```python
from build123d import *

# Parameters (mm, degrees)
BOSS_EXTRUDE3_DEPTH = 150
SKETCH3_W           = 5
SKETCH3_H           = 300
BOSS_EXTRUDE4_DEPTH = 194.04


with BuildPart() as part:
    # Sketch1 → Boss-Extrude3 (new, symmetric)
    with BuildSketch(Plane.XY):
        Polygon((-605.658970563, 869.326926327), (-605.421491465, 714.331361266), (-602.421487943, 714.331361266), (-602.651320044, 864.335957761), (-602.656320364, 867.599518288), (-455.616774381, 952.797835671), (-452.784185512, 951.168221277), (-322.765615027, 876.367343414), (-321.26959747, 878.967714824), (-451.288167955, 953.768592687), (-455.622120304, 956.261955282), align=None)
    extrude(amount=BOSS_EXTRUDE3_DEPTH, both=True)

    # Sketch3 → Boss-Extrude4 (add)
    with BuildSketch(Plane(origin=(-529.334093448, 913.551431111, 0), x_dir=(0.8652472150761933, 0.5013454465764019, 0), z_dir=(-0.5013454465764018, 0.8652472150761932, 0))):
        with Locations((62.691806295, 0)):
            Rectangle(SKETCH3_W, SKETCH3_H)
        with Locations((-65.711641465, 0)):
            Rectangle(SKETCH3_W, SKETCH3_H)
    extrude(amount=BOSS_EXTRUDE4_DEPTH)


solid = part.part
```
Design review of the part built by this model. Coordinates are the model's own, in mm. A direction names the side the tool comes from. Coordinates: 2 decimals unless noted, no trailing zeros. Loops run counter-clockwise (first coordinate to the right, second up) from the corner with the lowest first, then second, coordinate; pieces in that order, holes last.
Q1. We need section B-B on y = 1041. State the section outline as (x, z) points.
Reported:
outline: (-682.02, -150) - (-676.24, -150) - (-676.24, 150) - (-682.02, 150) - close; (-533.61, -150) - (-527.84, -150) - (-527.84, 150) - (-533.61, 150) - close
Q2. For pin 1 (2 mm diameter, centred on x = -376.5, z = 101, fed in from -Y); pin 2 (10 mm diameter, centred on y = 1010.5, z = -65.5, fed in from -X); pin 3 (10 mm diameter, centred on y = 1002.5, z = -29, fed in from -X), all flat-tipped, find the tip position at first contact; note any pin that passes through.
Reported:
pin 1: stops at y = 906.71
pin 2: stops at x = -667.24
pin 3: stops at x = -662.61
Q3. To check wall thickness, follow line 1 (X direction, y = 902, z = -90); line 2 (X direction, y = 909.5, z = 130); line 3 (Y direction, x = -488, z = 42). State the ranges of each line that lie inside material, in increasing order.
Reported:
line 1: x = -601.48 to -595.7, -549.27 to -543.29, -367.32 to -361.3
line 2: x = -605.82 to -600.04, -536.33 to -530.34, -380.36 to -374.34
line 3: y = 934.03 to 937.5, 962.28 to 972.25
Q4. Tool access review of faces 1 (the face through (-596.9, 874.4, 2.1)), 2 (the face through (-529.89, 913.23, 2.1)), 3 (the face through (-530.17, 909.6, 2.1)): name each direction out of +Z, -Z, +X, -X, +Y, -Y from which nothing blocks a thin tool from reaching the whole face with its end or side.
Reported:
face 1: +Z, -Z, -X
face 2: +Z, -Z
face 3: +Z, -Z, -Y
Q5. We need section D-D on x = -429.5. State the section outline as (y, z) points.
Reported:
outline: (937.77, -150) - (941.23, -150) - (941.23, 150) - (937.77, 150) - close
Q6. We need section C-C on z = -81. State the section outline as (x, y) points.
Reported:
outline: (-685.64, 1047.25) - (-588.35, 879.35) - (-605.66, 869.33) - (-605.42, 714.33) - (-602.42, 714.33) - (-602.66, 867.6) - (-455.62, 952.8) - (-322.77, 876.37) - (-321.27, 878.97) - (-455.62, 956.26) - (-472.93, 946.24) - (-570.21, 1114.13) - (-574.53, 1111.62) - (-477.25, 943.73) - (-584.03, 881.86) - (-681.31, 1049.75) - close
Q7. The part is to be moulded in two halves that separate along X. For faces 4 (the face through (-518, 1019, -150)), 5 (the face through (-636.3, 962.1, 2.1)), 6 (the face through (-631.987, 964.632, 2.1)), say which applies: +X half, -X half, draft (parallel to the pull), parting line (faces both ways), or undercut.
Reported:
face 4: draft
face 5: -X half
face 6: undercut
Q8. We need section A-A on x = -525. State the section outline as (y, z) points, and give its area (3 significant figures).
Reported:
outline: (912.6, -150) - (916.06, -150) - (916.06, 150) - (912.6, 150) - close; (1026.13, -150) - (1036.11, -150) - (1036.11, 150) - (1026.13, 150) - close
area: 4,030 mm2
